```python
from build123d import *


with BuildPart() as f1:
    # F0 (on Front) → F1 (revolve)
    with BuildSketch(Plane.XZ):
        with BuildLine():
            Line((-126.587485, 0), (0, 0))
            Line((0, 0), (0, 50))
            Line((0, 50), (-86.60254, 200))
            Line((-86.60254, 200), (-156.60254, 200))
            Line((-156.60254, 200), (-156.60254, 150))
            Line((-156.60254, 150), (-276.463263, 150))
            Line((-276.463263, 150), (-279.444389, 150))
            ThreePointArc((-279.444389, 150), (-297.578514, 145.460746), (-315.712638, 150))
            Line((-315.712638, 150), (-356.60254, 150))
            Line((-356.60254, 150), (-376.587485, 130.015055))
            Line((-376.587485, 130.015055), (-376.587485, 70))
            Line((-376.587485, 70), (-276.587485, 70))
            Line((-276.587485, 70), (-276.587485, 50))
            Line((-276.587485, 50), (-126.587485, 50))
            Line((-126.587485, 50), (-126.587485, 0))
        make_face()
    revolve(axis=Axis((-63.293743, 0, 0), (1, 0, 0)))


solid = f1.part
```
Geometry check sheet. Reference: the model listing, model coordinates, mm. A direction names the side the tool comes from. Coordinates: 2 decimals unless noted, no trailing zeros. Order: outer loops, then holes, each group sorted by start corner. A loop starts at its lowest first (then second) coordinate and runs counter-clockwise, first axis right, second up.
Q1. Sectioned sample at A-A on y = 0. Record the cut outline in (x, z).
Reply:
outline: (-376.59, -130.02) - (-356.6, -150) - (-315.71, -150) arc R38.49 cw to (-279.44, -150) - (-156.6, -150) - (-156.6, -200) - (-86.6, -200) - (0, -50) - (0, 50) - (-86.6, 200) - (-156.6, 200) - (-156.6, 150) - (-279.44, 150) arc R38.49 cw to (-315.71, 150) - (-356.6, 150) - (-376.59, 130.02) - (-376.59, 70) - (-276.59, 70) - (-276.59, 50) - (-126.59, 50) - (-126.59, -50) - (-276.59, -50) - (-276.59, -70) - (-376.59, -70) - close
Q2. Draft check along Z on faces 1 (the face through (-375.617, -39.344, 124.937)), 2 (the face through (-126.587, -1, -1)), 3 (the face through (-200.54, -15.02, 47.69)), 4 (the face through (-376.587, 56, 56)). Enter one of: released by +Z, released by -Z, zero draft, split by the parting line, or undercut.
Reply:
face 1: split by the parting line
face 2: undercut
face 3: undercut
face 4: zero draft
Q3. Tool access check on faces 5 (the face through (-5.417, 57.971, -12.873)), 6 (the face through (-276.587, -17, -48)). Record the directions out of +Z, -Z, +X, -X, +Y, -Y that give a thin tool (end or side, any length) a straight path to the whole face; none if there is none.
Reply:
face 5: +X
face 6: -X
Q4. Sectioned sample at D-D on x = -30.5. Record the cut outline in (y, z).
Reply:
outline: circle Ø205.66 at (0, 0)
Q5. Sectioned sample at C-C on x = -212.5. Record the cut outline in (y, z), and give its area (3 significant figures).
Reply:
outline: circle Ø300 at (0, 0); hole circle Ø100 at (0, 0)
area: 62,800 mm2
Q6. Thickness scan on probe 1 along Y at (x, z) = (-326, 0); probe 2 along Y at (x, z) = (-315.5, 0). Record the ranges inside material, lowest first.
Reply:
probe 1: y = -150 to -70, 70 to 150
probe 2: y = -149.89 to -70, 70 to 149.89
Q7. Depth check by flat-ended pin: pin 1 Ø5 at (y, z) = (-89, 110) entering from -X; pin 2 Ø4 at (x, z) = (-301.5, 70.5) entering from -Y; pin 3 Ø10 at (x, z) = (-110.5, -150.5) entering from +Y. Enter the tip coordinate at first touch or a pass-through.
Reply:
pin 1: stops at x = -367.61
pin 2: stops at y = -128.58
pin 3: stops at y = 137.22
